from build123d import *

# Parameters (mm, degrees)
SKETCH1_W               = 184
SKETCH1_H               = 25
BOSS_EXTRUDE1_DEPTH     = 25
CUT_EXTRUDE1_DEPTH      = 97.234200727
CUT_EXTRUDE1_DEPTH_BACK = 97.234200727
SKETCH2_R               = 7.5


with BuildPart() as part:
    # Sketch1 → Boss-Extrude1 (new body)
    with BuildSketch(Plane.XY):
        with Locations((0, 0.615692496)):
            Rectangle(SKETCH1_W, SKETCH1_H)
    extrude(amount=BOSS_EXTRUDE1_DEPTH)

    # Sketch2 → Cut-Extrude1 (cut, two sides: drawn at the far end of the back side and taken through both)
    with BuildSketch(Plane.XY.offset(25).offset(-CUT_EXTRUDE1_DEPTH_BACK)):
        with Locations((-72, 0)):
            Circle(SKETCH2_R)
        with Locations((72, 0)):
            Circle(SKETCH2_R)
    extrude(amount=CUT_EXTRUDE1_DEPTH + CUT_EXTRUDE1_DEPTH_BACK, mode=Mode.SUBTRACT)


solid = part.part
Input: part model. Units: mm. Frame: model coordinates. Coordinates: 2 decimals unless noted, no trailing zeros. Loops run counter-clockwise (first coordinate to the right, second up) from the corner with the lowest first, then second, coordinate; pieces in that order, holes last.
(1) Material intervals for probe 1 along X at (y, z) = (0, 7.75); probe 2 along Y at (x, z) = (-72, 15); probe 3 along X at (y, z) = (4.5, 10.5), sorted ascending.
(2) Section B-B on x = 72. Return the cut outline in (y, z), then the cut area to 3 significant figures.
(3) Pull-direction query (Y, two-part tool) for faces 1 (the face through (64.507, 0.33, 12.325)), 2 (the face through (92, 0, 12)), 3 (the face through (-1, -11.884, 12)); classes: released by +Y, released by -Y, zero draft, split by the parting line, or undercut.
(4) Section C-C on z = 10.75. Return the cut outline in (x, y), then the cut area to 3 significant figures.
(5) Section A-A on y = 0. Return the cut outline in (x, z), then the cut area to 3 significant figures.
(6) First-contact query: pin 1 Ø5 at (x, y) = (48.5, 2) entering from -Z. Flat tip, straight axial feed; report the tip coordinate or a pass-through.
Data:
1. probe 1: x = -92 to -79.5, -64.5 to 64.5, 79.5 to 92
1. probe 2: y = -11.88 to -7.5, 7.5 to 13.12
1. probe 3: x = -92 to -78, -66 to 66, 78 to 92
2. outline: (-11.88, 0) - (-7.5, 0) - (-7.5, 25) - (-11.88, 25) - close; (7.5, 0) - (13.12, 0) - (13.12, 25) - (7.5, 25) - close
2. area: 250 mm2
3. face 1: undercut
3. face 2: zero draft
3. face 3: released by -Y
4. outline: (-92, -11.88) - (92, -11.88) - (92, 13.12) - (-92, 13.12) - close; hole circle Ø15 at (-72, 0); hole circle Ø15 at (72, 0)
4. area: 4,250 mm2
5. outline: (-92, 0) - (-79.5, 0) - (-79.5, 25) - (-92, 25) - close; (-64.5, 0) - (64.5, 0) - (64.5, 25) - (-64.5, 25) - close; (79.5, 0) - (92, 0) - (92, 25) - (79.5, 25) - close
5. area: 3,850 mm2
6. pin 1: stops at z = 0
